Read the model definition and answer for the solid it produces. Units are mm, in the model's axes. Face numbers are marked on the shaded views. A direction names the side the tool comes from. Give positions to 0.01 mm unless a question says otherwise; leave off trailing zeros. Write each loop counter-clockwise with the first axis right and the second up, starting at its lowest first coordinate (ties: lowest second). Pieces come first, ordered by that corner, then holes.
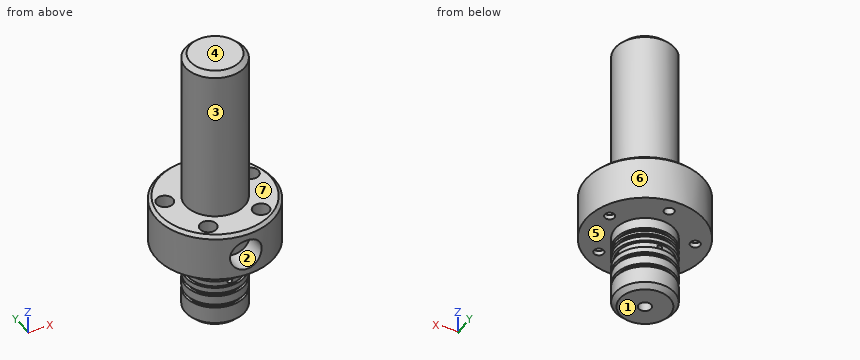
```python
from build123d import *

# Parameters (mm, degrees)
SKETCH1_R                 = 18.875
BOSS_EXTRUDE1_DEPTH       = 47.85
SKETCH2_R                 = 37.5
BOSS_EXTRUDE2_DEPTH       = 30
SKETCH11_R                = 3.125
CUT_EXTRUDE4_DEPTH        = 30
SKETCH12_R                = 4.7625
CUT_EXTRUDE5_DEPTH        = 8
SKETCH13_W                = 2.1
SKETCH13_H                = 3
SKETCH13_W_2              = 4.5
SKETCH13_H_2              = 2.2
SKETCH18_R                = 3.125
CUT_EXTRUDE8_DEPTH        = 30
SKETCH19_R                = 5.25
CUT_EXTRUDE9_DEPTH        = 27
CHAMFER1_SIZE             = 2
SKETCH20_R                = 18.875
BOSS_EXTRUDE3_DEPTH       = 100
F_8_0MM_DOWEL_HOLE1_D     = 8
F_8_0MM_DOWEL_HOLE1_DEPTH = 77.85
F_8_0MM_DOWEL_HOLE1_TIP   = 2.403442476
CHAMFER2_SIZE             = 3
SKETCH26_R                = 1.5
CUT_EXTRUDE10_DEPTH       = 186.58858401
CIRPATTERN1_COUNT         = 4


with BuildPart() as part:
    # Sketch1 → Boss-Extrude1 (new body)
    with BuildSketch(Plane.XY):
        Circle(SKETCH1_R)
    extrude(amount=BOSS_EXTRUDE1_DEPTH)

    # Sketch2 → Boss-Extrude2 (add)
    with BuildSketch(Plane.XY.offset(47.85)):
        Circle(SKETCH2_R)
    extrude(amount=BOSS_EXTRUDE2_DEPTH)

    # Sketch11 → Cut-Extrude4 (cut)
    with BuildSketch(Plane.XY.offset(77.85)):
        with Locations((0, 28.5)):
            Circle(SKETCH11_R)
    extrude(amount=-CUT_EXTRUDE4_DEPTH, mode=Mode.SUBTRACT)

    # Sketch12 → Cut-Extrude5 (cut)
    with BuildSketch(Plane.XY.offset(77.85)):
        with Locations((0, 28.5)):
            Circle(SKETCH12_R)
    extrude(amount=-CUT_EXTRUDE5_DEPTH, mode=Mode.SUBTRACT)

    # Sketch13 → Cut-Revolve1 (revolve, cut)
    with BuildSketch(Plane(origin=(0, 0, 0), x_dir=(0, 0, -1), z_dir=(1, 0, 0)), mode=Mode.PRIVATE) as cut_revolve1_sk:
        with Locations((-14.85, 18.875)):
            Rectangle(SKETCH13_W, SKETCH13_H)
        with Locations((-22.85, 18.875)):
            Rectangle(SKETCH13_W, SKETCH13_H)
        with Locations((-35.85, 18.875)):
            Rectangle(SKETCH13_W, SKETCH13_H)
        with Locations((-39.85, 18.875)):
            Rectangle(SKETCH13_W, SKETCH13_H)
        with Locations((-29.85, 18.475)):
            Rectangle(SKETCH13_W_2, SKETCH13_H_2)
    revolve(cut_revolve1_sk.sketch.rotate(Axis((0, 0, 0), (0, 0, 1)), 90), axis=Axis((0, 0, 0), (0, 0, 1)), mode=Mode.SUBTRACT)

    # Sketch18 → Cut-Extrude8 (cut)
    with BuildSketch(Plane.XY.offset(77.85)):
        with Locations((27.105110714, 8.80698434)):
            Circle(SKETCH18_R)
        with Locations((16.75187969, -23.05698434)):
            Circle(SKETCH18_R)
        with Locations((-16.75187969, -23.05698434)):
            Circle(SKETCH18_R)
        with Locations((-27.105110714, 8.80698434)):
            Circle(SKETCH18_R)
    extrude(amount=-CUT_EXTRUDE8_DEPTH, mode=Mode.SUBTRACT)

    # Sketch19 → Cut-Extrude9 (cut)
    with BuildSketch(Plane.XY.offset(77.85)):
        with Locations((27.105110714, 8.80698434)):
            Circle(SKETCH19_R)
        with Locations((16.75187969, -23.05698434)):
            Circle(SKETCH19_R)
        with Locations((-16.75187969, -23.05698434)):
            Circle(SKETCH19_R)
        with Locations((-27.105110714, 8.80698434)):
            Circle(SKETCH19_R)
    extrude(amount=-CUT_EXTRUDE9_DEPTH, mode=Mode.SUBTRACT)

    # Chamfer1
    chamfer1_edges = [part.edges().sort_by_distance(p)[0] for p in [
        (-37.5, 0, 77.85),
    ]]
    chamfer(chamfer1_edges, length=CHAMFER1_SIZE)

    # Sketch20 → Boss-Extrude3 (add)
    with BuildSketch(Plane.XY.offset(77.85)):
        with Locations(Location((0, 0, 0), (0, 0, 180))):
            Circle(SKETCH20_R)
    extrude(amount=BOSS_EXTRUDE3_DEPTH)

    # Ø8.0mm Dowel Hole1
    with Locations(Plane(origin=(0, 0, 0), x_dir=(-1, 0, 0), z_dir=(0, 0, -1))):
        with Locations((0, 0)):
            Hole(F_8_0MM_DOWEL_HOLE1_D / 2, depth=F_8_0MM_DOWEL_HOLE1_DEPTH)
            with Locations((0, 0, -(F_8_0MM_DOWEL_HOLE1_DEPTH + F_8_0MM_DOWEL_HOLE1_TIP / 2))):  # 118° drill point
                Cone(0, F_8_0MM_DOWEL_HOLE1_D / 2, F_8_0MM_DOWEL_HOLE1_TIP, mode=Mode.SUBTRACT)

    # Sketch25 → Cut-Revolve2 (revolve, cut)
    with BuildSketch(Plane(origin=(0, 0, 0), x_dir=(0, 0, -1), z_dir=(1, 0, 0))):
        Polygon((-65.25, 0), (-65.25, -12.5), (-65.85, -12.5), (-65.85, -22.5), (-71.85, -22.5), (-71.85, -41.115481675), (-61.85, -41.115481675), (-61.85, 0), align=None)
    revolve(axis=Axis((0, 37.5, 61.85), (0, -1, 0)), mode=Mode.SUBTRACT)

    # Chamfer2
    chamfer2_edges = [part.edges().sort_by_distance(p)[0] for p in [
        (18.875, 0, 177.85),
        (-18.875, 0, 0),
    ]]
    chamfer(chamfer2_edges, length=CHAMFER2_SIZE)

    # Sketch26 → Cut-Extrude10 (cut, through all)
    with BuildSketch(Plane(origin=(0, 0, 0), x_dir=(1, 0, 0), z_dir=(0, 1, 0))):
        with Locations(Location((0, -29.85, 0), (0, 0, 270))):
            Circle(SKETCH26_R)
    cut_extrude10 = extrude(amount=-CUT_EXTRUDE10_DEPTH, mode=Mode.SUBTRACT)

    # CirPattern1: Cut-Extrude10 ×4 about axis
    cirpattern1_axis = Axis((0, 0, 27.6), (0, 0, -1))
    for i in range(1, CIRPATTERN1_COUNT):
        add(cut_extrude10.rotate(cirpattern1_axis, i * 360 / CIRPATTERN1_COUNT), mode=Mode.SUBTRACT)


solid = part.part
```
Item 1: Each of these flat-tipped pins is pushed along its axis until it touches: pin 1 Ø8 at (x, z) = (-2, 157.5) entering from +Y (3 decimals); pin 2 Ø8.5 at (x, y) = (28, 10) entering from +Z; pin 3 Ø6 at (x, z) = (4, 26) entering from +Y. Where does it stop, or does it pass through?
Result set:
pin 1: stops at y = 18.875
pin 2: stops at z = 77.85
pin 3: stops at y = 18.85
Item 2: Determine the mould class of the marked faces 1, 2, 3 and 4 for opening direction Z: pulls with the +Z half, pulls with the -Z half, needs draft (parallel to the pull), parting line crosses it, or undercut.
Result set:
face 1: pulls with the -Z half
face 2: undercut
face 3: needs draft
face 4: pulls with the +Z half
Item 3: Section C-C (z = 61.85) is taken. Write down the section's boundary in (x, y) (3 decimals), and give its area (3 significant figures).
Result set:
outline: (-10, -36.142) - (-10, -22.5) - (-4, -22.5) - (-4, -12.5) - (-3.4, -12.5) - (-3.4, -2.107) arc R4 cw (long way) to (3.4, -2.107) - (3.4, -12.5) - (4, -12.5) - (4, -22.5) - (10, -22.5) - (10, -36.142) arc R37.5 ccw (long way) to start; hole circle Ø10.5 at (-27.105, 8.807); hole circle Ø10.5 at (-16.752, -23.057); hole circle Ø6.25 at (0, 28.5); hole circle Ø10.5 at (16.752, -23.057); hole circle Ø10.5 at (27.105, 8.807)
area: 3,560 mm2
Item 4: Find the intervals of material crossed by line 1 along X through (y, z) = (8, 62); line 2 along Z through (x, y) = (0, -5.5); line 3 along Z through (x, y) = (0, 14.5), in increasing order.
Result set:
line 1: x = -36.64 to -32.29, -21.92 to 21.92, 32.29 to 36.64
line 2: z = 0 to 28.35, 31.35 to 58.45, 65.25 to 177.85
line 3: z = 0 to 28.35, 31.35 to 177.85
Item 5: Section A-A (z = 89.5) is taken. Write down the section's boundary in (x, y) (3 decimals).
Result set:
outline: circle Ø37.75 at (0, 0)
Item 6: Section B-B (z = 11.5) is taken. Write down the section's boundary in (x, y) (3 decimals), and give its area (3 significant figures).
Result set:
outline: circle Ø37.75 at (0, 0); hole circle Ø8 at (0, 0)
area: 1,070 mm2
Item 7: Which of the six approach directions +Z, -Z, +X, -X, +Y, -Y give full straight-line access (tool end or side, diameter ignored) to the marked faces 5, 6 and 7?
Result set:
face 5: -Z
face 6: +Z, -Z
face 7: +Z
